```python
from build123d import *

# Parameters (mm, degrees)
SKETCH1_W            = 304.8
SKETCH1_H            = 304.8
BOSS_EXTRUDE1_DEPTH  = 5.08
SKETCH2_W            = 25.4
SKETCH2_H            = 25.4
CUT_EXTRUDE1_DEPTH   = 5.08
LPATTERN1_COUNT      = 3
LPATTERN1_PITCH      = 76.2
LPATTERN1_COUNT_DIR2 = 2
LPATTERN1_PITCH_DIR2 = 101.6
SKETCH3_W            = 25.4
SKETCH3_H            = 50.8
CUT_EXTRUDE2_DEPTH   = 7.62


with BuildPart() as part:
    # Sketch1 → Boss-Extrude1 (new body)
    with BuildSketch(Plane(origin=(0, 0, 0), x_dir=(1, 0, 0), z_dir=(0, 1, 0))):
        Rectangle(SKETCH1_W, SKETCH1_H)
    extrude(amount=BOSS_EXTRUDE1_DEPTH)

    # Sketch2 → Cut-Extrude1 (cut)
    with BuildSketch(Plane(origin=(0, 5.08, 0), x_dir=(1, 0, 0), z_dir=(0, 1, 0))):
        with Locations((-12.7, 88.9)):
            Rectangle(SKETCH2_W, SKETCH2_H)
    cut_extrude1 = extrude(amount=-CUT_EXTRUDE1_DEPTH, mode=Mode.SUBTRACT)

    # LPattern1: Cut-Extrude1 3 × 2
    with Locations(*[(j * LPATTERN1_PITCH_DIR2, 0, i * LPATTERN1_PITCH) for i in range(LPATTERN1_COUNT) for j in range(LPATTERN1_COUNT_DIR2) if (i, j) != (0, 0)]):
        add(cut_extrude1, mode=Mode.SUBTRACT)

    # Sketch3 → Cut-Extrude2 (cut)
    with BuildSketch(Plane(origin=(0, 5.08, 0), x_dir=(1, 0, 0), z_dir=(0, 1, 0))):
        with Locations((-91.407513773, 51.049523057)):
            Rectangle(SKETCH3_W, SKETCH3_H)
    extrude(amount=-CUT_EXTRUDE2_DEPTH, mode=Mode.SUBTRACT)


solid = part.part
```
Read the model definition and answer for the solid it produces. Units are mm, in the model's axes. Give positions to 0.01 mm unless a question says otherwise; leave off trailing zeros. Loops run counter-clockwise (first coordinate to the right, second up) from the corner with the lowest first, then second, coordinate; pieces in that order, holes last.
Item 1: The part is cut by section C-C (x = -8). Write down the section's boundary in (y, z).
Item 2: Find the intervals of material crossed by line 1 along Z through (x, y) = (-2, 0.3); line 2 along X through (y, z) = (0.2, -96); line 3 along Z through (x, y) = (-91.5, 0.4), in increasing order.
Item 3: The part is cut by section A-A (z = -92.5). Write down the section's boundary in (x, y), and give its area (3 significant figures).
Item 4: The part is cut by section B-B (y = 3.9). Give the number of separate pieces and of enclosed holes in the cut face, and give its area (3 significant figures).
Item 5: The part is cut by section D-D (z = -48). Write down the section's boundary in (x, y), and give its area (3 significant figures).
Taken from the geometry:
1. outline: (0, -152.4) - (5.08, -152.4) - (5.08, -101.6) - (0, -101.6) - close; (0, -76.2) - (5.08, -76.2) - (5.08, -25.4) - (0, -25.4) - close; (0, 0) - (5.08, 0) - (5.08, 50.8) - (0, 50.8) - close; (0, 76.2) - (5.08, 76.2) - (5.08, 152.4) - (0, 152.4) - close
2. line 1: z = -152.4 to -101.6, -76.2 to -25.4, 0 to 50.8, 76.2 to 152.4
2. line 2: x = -152.4 to -25.4, 0 to 76.2, 101.6 to 152.4
2. line 3: z = -152.4 to -76.45, -25.65 to 152.4
3. outline: (-152.4, 0) - (-25.4, 0) - (-25.4, 5.08) - (-152.4, 5.08) - close; (0, 0) - (76.2, 0) - (76.2, 5.08) - (0, 5.08) - close; (101.6, 0) - (152.4, 0) - (152.4, 5.08) - (101.6, 5.08) - close
3. area: 1,290 mm2
4. separate pieces: 1
4. enclosed holes: 7
4. area: 87,700 mm2
5. outline: (-152.4, 0) - (-104.11, 0) - (-104.11, 5.08) - (-152.4, 5.08) - close; (-78.71, 0) - (152.4, 0) - (152.4, 5.08) - (-78.71, 5.08) - close
5. area: 1,420 mm2
